The drawing under review shows one solid part. Ordinate dimensions are in mm from its lowest x, y, z. Coordinates: 2 decimals unless noted, no trailing zeros. Order: outer loops, then holes, each group sorted by start corner. A loop starts at its lowest first (then second) coordinate and runs counter-clockwise, first axis right, second up. Notation, with made-up numbers: (40, 64.5) - (53, 64.5) arc R8 cw to (53, 75.5) - close; hole circle Ø10 at (-12, 61.25). An arc over 180 degrees is marked (long way). Answer in a Markdown table with one row per item.
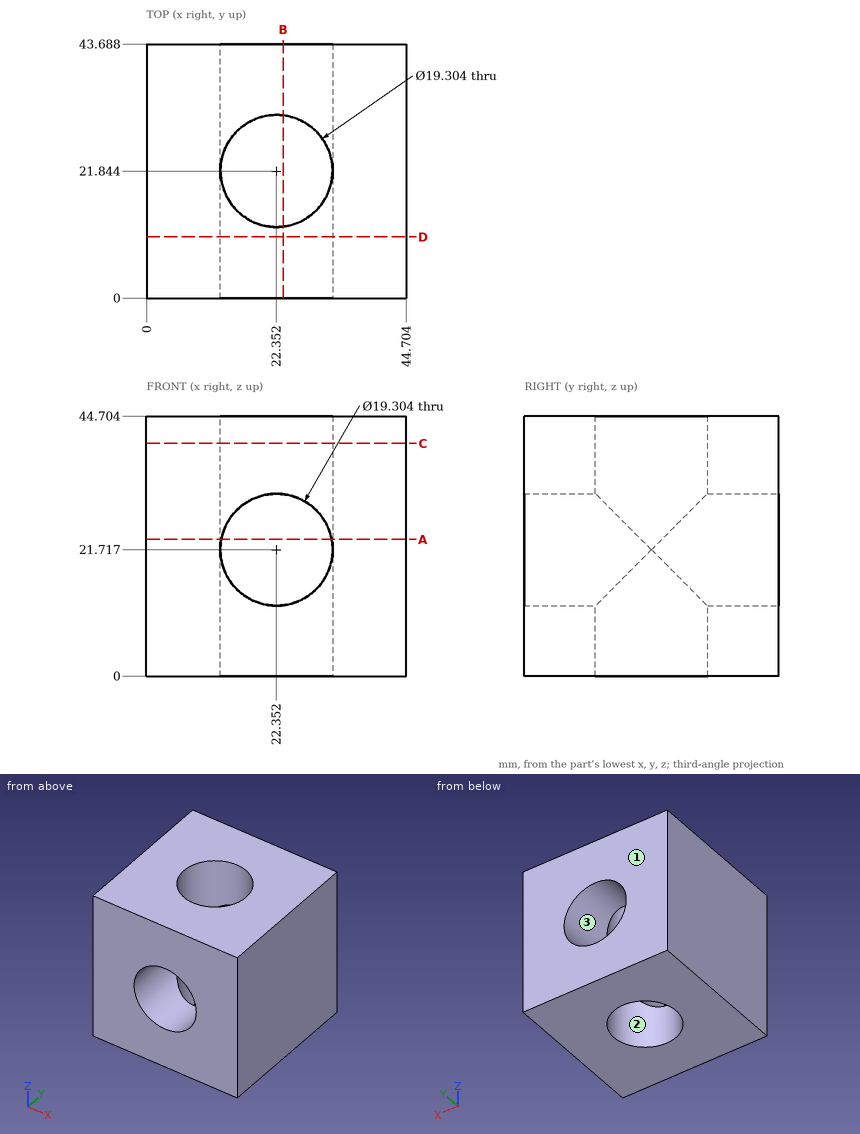
Item 1: We need section B-B, the plane x = 23.5. Write out the cut boundary in (y, z).
Check values:
| item | result |
|---|---|
| outline | (0, 0) - (12.26, 0) - (12.26, 12.13) - (0, 12.13) - close; (0, 31.3) - (12.26, 31.3) - (12.26, 44.7) - (0, 44.7) - close; (31.43, 0) - (43.69, 0) - (43.69, 12.13) - (31.43, 12.13) - close; (31.43, 31.3) - (43.69, 31.3) - (43.69, 44.7) - (31.43, 44.7) - close |
Item 2: To check wall thickness, follow line 1 (Y direction, x = 17, z = 38); line 2 (X direction, y = 21, z = 36); line 3 (X direction, y = 24.5, z = 5). State the ranges of each line that lie inside material, in increasing order. Write a range as from..to.
Check values:
| item | result |
|---|---|
| line 1 | 0..13.81, 29.88..43.69 |
| line 2 | 0..12.74, 31.97..44.7 |
| line 3 | 0..13.07, 31.63..44.7 |
Item 3: Mouldability with a two-part tool opening along Y and no side actions: class the marked faces 1, 2 and 3 as +Y half, -Y half, draft (parallel to the pull), parting line (faces both ways), or undercut.
Check values:
| item | result |
|---|---|
| face 1 | +Y half |
| face 2 | undercut |
| face 3 | draft |
Item 4: Clearance check with a flat-ended pin moving along its axis: pin 1 Ø2 at (y, z) = (23, 10) entering from -X. State where the tip first meets the part, or that it passes through.
Check values:
| item | result |
|---|---|
| pin 1 | x = 0 |
Item 5: We need section D-D, the plane y = 10.5. Write out the cut boundary in (x, z), then the cut area to 3 significant figures.
Check values:
| item | result |
|---|---|
| outline | (0, 0) - (44.7, 0) - (44.7, 44.7) - (0, 44.7) - close; hole circle Ø19.3 at (22.35, 21.72) |
| area | 1,710 mm^2 |
Item 6: We need section A-A, the plane z = 23.5. Write out the cut boundary in (x, y), then the cut area to 3 significant figures.
Check values:
| item | result |
|---|---|
| outline | (0, 0) - (12.87, 0) - (12.87, 20.06) arc R9.65 cw to (12.87, 23.63) - (12.87, 43.69) - (0, 43.69) - close; (31.84, 0) - (44.7, 0) - (44.7, 43.69) - (31.84, 43.69) - (31.84, 23.63) arc R9.65 cw to (31.84, 20.06) - close |
| area | 1,120 mm^2 |
Item 7: We need section C-C, the plane z = 40. Write out the cut boundary in (x, y), then the cut area to 3 significant figures.
Check values:
| item | result |
|---|---|
| outline | (0, 0) - (44.7, 0) - (44.7, 43.69) - (0, 43.69) - close; hole circle Ø19.3 at (22.35, 21.84) |
| area | 1,660 mm^2 |
